Job drawing, mm, ordinate dimensions from the low corner. One solid piece. A direction names the side the tool comes from. Give positions to 0.01 mm unless a question says otherwise; leave off trailing zeros. Write each loop counter-clockwise with the first axis right and the second up, starting at its lowest first coordinate (ties: lowest second). Pieces come first, ordered by that corner, then holes. Notation, with made-up numbers: M -31,4 L -7,4 A17 ccw -7,15 Z; hole C -34.75,89.25 d3. An arc over 180 degrees is marked long. Answer as CSV lines item,"result". Start each with the question number.
Item 1: Wall check: L1, parallel to X at y = 17.5, z = 13; L2, parallel to X at y = 24.5, z = 20; L3, parallel to Z at x = 7.5, y = 20.5. Give the ranges that are in metal, low to high. Write a range as from..to.
Item 2: Two-plate mould, pull along X, no slides. Class the marked faces 1, 2 and 3: +X half, -X half, draft (parallel to the pull), parting line (faces both ways), or undercut.
Item 3: Pin check, flat tips, straight feed: pin 1 (4.5 mm diameter, centred on x = 3, z = 17.5, fed in from -Y); pin 2 (1 mm diameter, centred on y = 27, z = 20, fed in from -X); pin 3 (4.5 mm diameter, centred on x = 5, y = 19.5, fed in from +Z). Stop position of each tip, or through.
Item 4: Band-saw the part on D-D, the plane x = 22. List the corners of the cut face in (y, z), then the cut area to 3 significant figures.
Item 5: 3-axis set-ups, long thin cutter, end or side, ignore diameter. For the marked faces 4, 5 and 6: which of +Z, -Z, +X, -X, +Y, -Y reach the whole face in a straight line?
Item 6: Band-saw the part on B-B, the plane y = 22.5. List the corners of the cut face in (x, z), then the cut area to 3 significant figures.
Item 7: Band-saw the part on C-C, the plane z = 19. List the corners of the cut face in (x, y), then the cut area to 3 significant figures.
Item 8: Band-saw the part on A-A, the plane z = 23. List the corners of the cut face in (x, y).
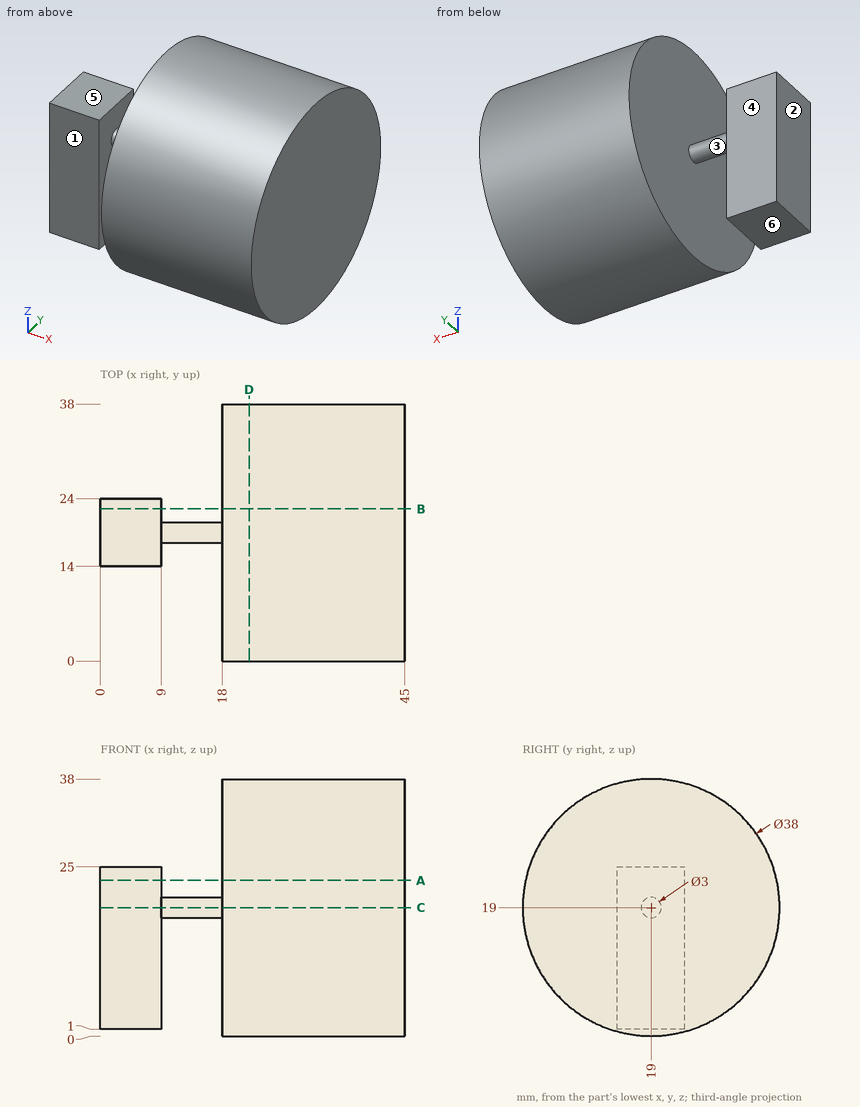
Output:
1,L1,"0..9, 18..45"
1,L2,"18..45"
1,L3,"1..25"
2,face 1,"draft"
2,face 2,"-X half"
2,face 3,"undercut"
3,pin 1,"y = 14"
3,pin 2,"x = 18"
3,pin 3,"z = 25"
4,outline,"C 19,19 d38"
4,area,"1,130 mm²"
5,face 4,"+Z, -Z, -X, +Y"
5,face 5,"+Z, -X, +Y, -Y"
5,face 6,"-Z, -X, +Y, -Y"
6,outline,"M 0,1 L 9,1 L 9,25 L 0,25 Z; M 18,0.33 L 45,0.33 L 45,37.67 L 18,37.67 Z"
6,area,"1,220 mm²"
7,outline,"M 0,14 L 9,14 L 9,17.5 L 18,17.5 L 18,0 L 45,0 L 45,38 L 18,38 L 18,20.5 L 9,20.5 L 9,24 L 0,24 Z"
7,area,"1,140 mm²"
8,outline,"M 0,14 L 9,14 L 9,24 L 0,24 Z; M 18,0.43 L 45,0.43 L 45,37.57 L 18,37.57 Z"
